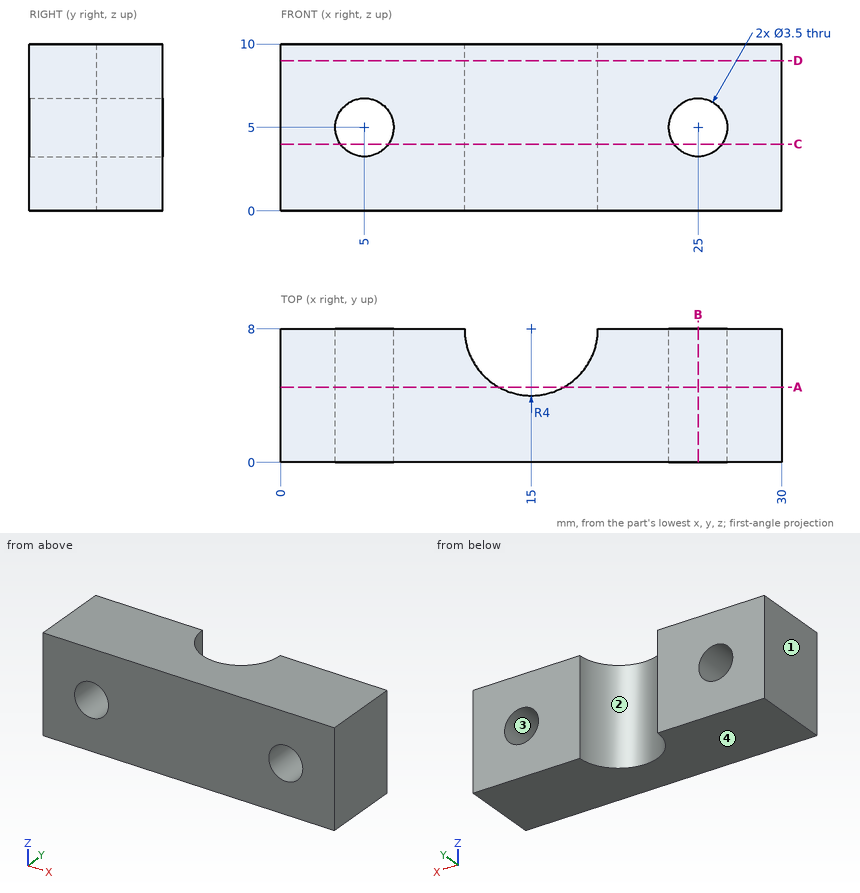
Can you work these out from the drawing? Everything is in mm from the part's minimum corner. Coordinates: 2 decimals unless noted, no trailing zeros. Write each loop counter-clockwise with the first axis right and the second up, starting at its lowest first coordinate (ties: lowest second). Pieces come first, ordered by that corner, then holes. Notation, with made-up numbers: (68, -9) -> (107, -9) arc R10 cw to (107, 2) -> close; hole circle Ø8 at (71, 70.5). An arc over 180 degrees is marked (long way). Write item = value, one per line.
(1) Imagine slicing it at B-B (x = 25). Please give me the cut outline in (y, z).
Verdict:
outline = (0, 0) -> (8, 0) -> (8, 3.25) -> (0, 3.25) -> close; (0, 6.75) -> (8, 6.75) -> (8, 10) -> (0, 10) -> close
(2) If I drill on probe 1 along X at (y, z) = (2, 5); probe 2 along X at (y, z) = (6, 5); probe 3 along X at (y, z) = (6.5, 4.25), over which ranges is the centre line in solid material (lowest first)?
Verdict:
probe_1 = 0 to 3.25, 6.75 to 23.25, 26.75 to 30
probe_2 = 0 to 3.25, 6.75 to 11.54, 18.46 to 23.25, 26.75 to 30
probe_3 = 0 to 3.42, 6.58 to 11.29, 18.71 to 23.42, 26.58 to 30
(3) Imagine slicing it at D-D (z = 9). Please give me the cut outline in (x, y).
Verdict:
outline = (0, 0) -> (30, 0) -> (30, 8) -> (19, 8) arc R4 cw to (11, 8) -> (0, 8) -> close
(4) Imagine slicing it at A-A (y = 4.5). Please give me the cut outline in (x, z), and give its area (3 significant figures).
Verdict:
outline = (0, 0) -> (13.06, 0) -> (13.06, 10) -> (0, 10) -> close; (16.94, 0) -> (30, 0) -> (30, 10) -> (16.94, 10) -> close; hole circle Ø3.5 at (5, 5); hole circle Ø3.5 at (25, 5)
area = 242 mm^2
(5) Thinking about a two-plate mould opening in X: for the marked faces 1, 2, 3 and 4, which applies, +X half, -X half, draft (parallel to the pull), parting line (faces both ways), or undercut?
Verdict:
face_1 = -X half
face_2 = undercut
face_3 = undercut
face_4 = draft
(6) Imagine slicing it at C-C (z = 4). Please give me the cut outline in (x, y).
Verdict:
outline = (0, 0) -> (3.56, 0) -> (3.56, 8) -> (0, 8) -> close; (6.44, 0) -> (23.56, 0) -> (23.56, 8) -> (19, 8) arc R4 cw to (11, 8) -> (6.44, 8) -> close; (26.44, 0) -> (30, 0) -> (30, 8) -> (26.44, 8) -> close
